The drawing under review shows one solid part. Ordinate dimensions are in mm from its lowest x, y, z. A direction names the side the tool comes from. Round coordinates to 2 decimals unless told otherwise and drop trailing zeros. Order: outer loops, then holes, each group sorted by start corner. A loop starts at its lowest first (then second) coordinate and runs counter-clockwise, first axis right, second up. Notation, with made-up numbers: (57, 53.25) -> (79, 53.25) arc R15 cw to (79, 64.25) -> close; hole circle Ø3 at (18.5, 75). An arc over 180 degrees is marked (long way). Use a Markdown table: item, result. Add a question column.
1) Wall thickness on line 1 along Y through (x, z) = (8, 5.25); line 2 along Z through (x, y) = (5.25, 2.5); line 3 along X through (y, z) = (9, 5.25): over which ranges is each line inside the solid? List them lowest first. Write a range as [from, to].
2) Draft analysis for pull direction X (two halves, no side actions). For the marked faces 3, 4 and 5, state which applies: pulls with the +X half, pulls with the -X half, needs draft (parallel to the pull), parting line crosses it, or undercut.
3) Clearance check with flat-ended pins moving along their axes: P1, Ø3, axis at y = 12, z = 3, coming from the -X side; P2, Ø5, axis at y = 14, z = 3, coming from the -X side. State where each tip first meets the part, or that it passes through.
4) Machinability: for the marked faces 1 and 2, which of the approach directions +Z, -Z, +X, -X, +Y, -Y give a long, thin tool a straight path to every point of the face, cutting with its end or side? Answer none if there is none.
5) Consider section D-D (y = 13.25). State the section outline as (x, z) points.
6) Consider section A-A (y = 8). State the section outline as (x, z) points.
7) Consider section C-C (z = 3.5). State the section outline as (x, y) points.
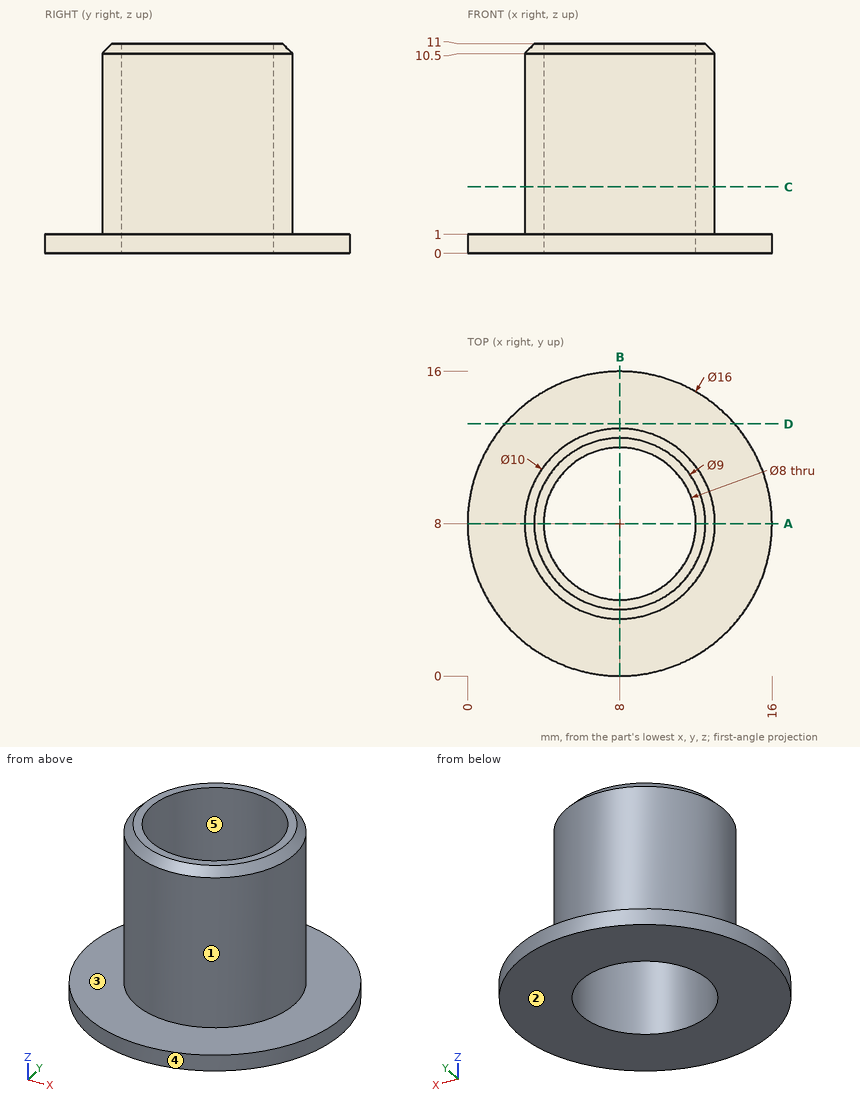
Results list:
| question | item | result |
|---|---|---|
| 1 | line 1 | [3, 4], [12, 13] |
| 1 | line 2 | [0, 1] |
| 1 | line 3 | [3.1, 4.13], [11.87, 12.9] |
| 2 | face 3 | needs draft |
| 2 | face 4 | parting line crosses it |
| 2 | face 5 | undercut |
| 3 | P1 | x = 3.67 |
| 3 | P2 | x = 1.39 |
| 4 | face 1 | +Z |
| 4 | face 2 | -Z, +X, -X, +Y, -Y |
| 5 | outline | (1.96, 0) -> (14.04, 0) -> (14.04, 1) -> (1.96, 1) -> close |
| 6 | outline | (0, 0) -> (4, 0) -> (4, 11) -> (3.5, 11) -> (3, 10.5) -> (3, 1) -> (0, 1) -> close; (12, 0) -> (16, 0) -> (16, 1) -> (13, 1) -> (13, 10.5) -> (12.5, 11) -> (12, 11) -> close |
| 7 | outline | circle Ø10 at (8, 8); hole circle Ø8 at (8, 8) |
